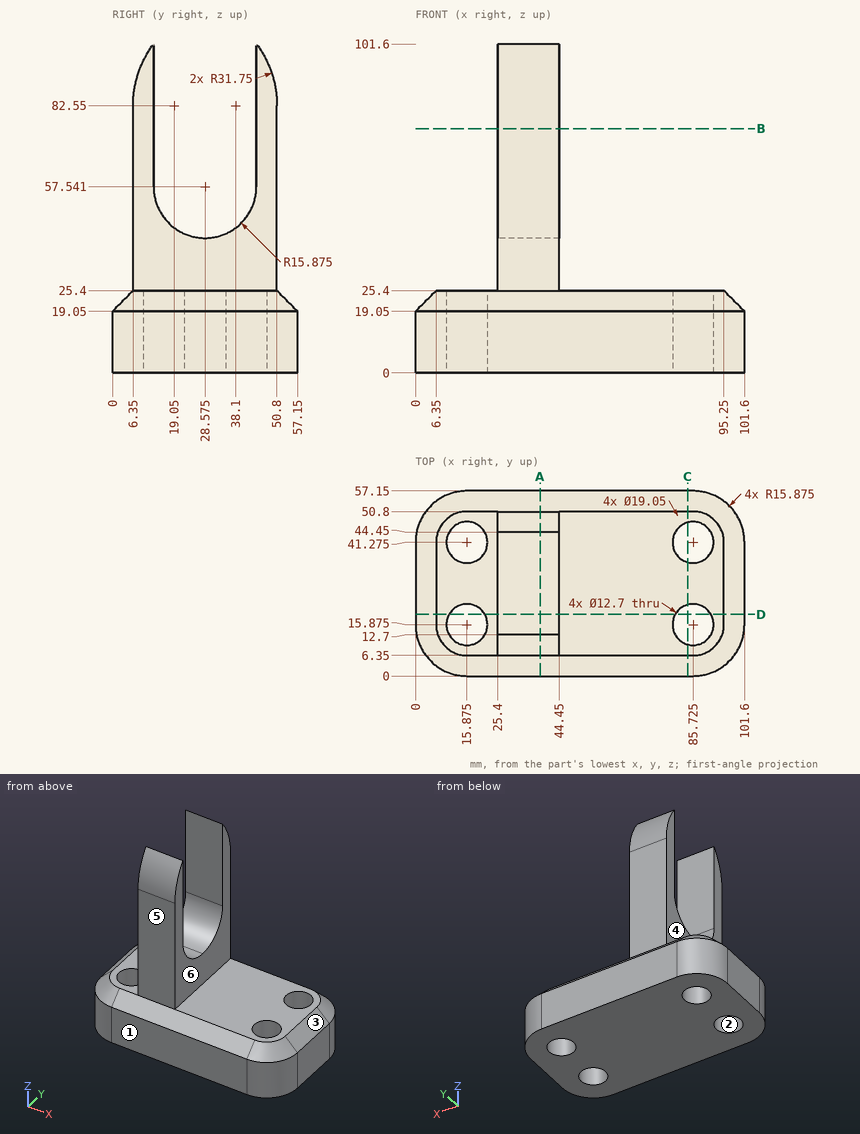
Can you work these out from the drawing? Everything is in mm from the part's minimum corner. A direction names the side the tool comes from. Round coordinates to 2 decimals unless told otherwise and drop trailing zeros. Write each loop counter-clockwise with the first axis right and the second up, starting at its lowest first coordinate (ties: lowest second). Pieces come first, ordered by that corner, then holes. Notation, with made-up numbers: M 87.5,64.5 L 93.5,64.5 A19 ccw 93.5,79.5 Z; hole C 24.5,59.25 d5. An arc over 180 degrees is marked long. Use a Markdown table: item, result.
Item 1: I want a section at B-B (z = 75.5). List the corners of the cut face in (x, y) for me.
Found:
| item | result |
|---|---|
| outline | M 25.4,6.35 L 44.45,6.35 L 44.45,12.7 L 25.4,12.7 Z; M 25.4,44.45 L 44.45,44.45 L 44.45,50.8 L 25.4,50.8 Z |
Item 2: I want a section at C-C (x = 84). List the corners of the cut face in (y, z) for me.
Found:
| item | result |
|---|---|
| outline | M 0,0 L 9.76,0 L 9.76,25.4 L 6.35,25.4 L 0,19.05 Z; M 21.99,0 L 35.16,0 L 35.16,25.4 L 21.99,25.4 Z; M 47.39,0 L 57.15,0 L 57.15,19.05 L 50.8,25.4 L 47.39,25.4 Z |
Item 3: We'd pull the mould along X, two halves only. Please class the marked faces 1, 2 and 3: released by +X, released by -X, zero draft, split by the parting line, or undercut.
Found:
| item | result |
|---|---|
| face 1 | zero draft |
| face 2 | undercut |
| face 3 | released by +X |
Item 4: I want a section at D-D (y = 19). List the corners of the cut face in (x, z) for me, and give its area (3 significant figures).
Found:
| item | result |
|---|---|
| outline | M 0,0 L 10.35,0 L 10.35,25.4 L 6.35,25.4 L 0,19.05 Z; M 21.4,0 L 80.2,0 L 80.2,25.4 L 44.45,25.4 L 44.45,44.88 L 25.4,44.88 L 25.4,25.4 L 21.4,25.4 Z; M 91.25,0 L 101.6,0 L 101.6,19.05 L 95.25,25.4 L 91.25,25.4 Z |
| area | 2,350 mm2 |
Item 5: I want a section at A-A (x = 38.5). List the corners of the cut face in (y, z) for me (3 decimals), and give its area (3 significant figures).
Found:
| item | result |
|---|---|
| outline | M 0,0 L 57.15,0 L 57.15,19.05 L 50.8,25.4 L 50.8,82.55 A31.75 ccw 44.45,101.6 L 44.45,57.541 A15.875 cw 12.7,57.541 L 12.7,101.6 A31.75 ccw 6.35,82.55 L 6.35,25.4 L 0,19.05 Z |
| area | 2,930 mm2 |
Item 6: If I drill on line 1 along X through (y, z) = (10, 36); line 2 along Z through (x, y) = (22.5, 31.5); line 3 along Y through (x, z) = (44, 75.5), over which ranges is the centre line in solid material (lowest first)? Write a range as [from, to].
Found:
| item | result |
|---|---|
| line 1 | x = [25.4, 44.45] |
| line 2 | z = [0, 25.4] |
| line 3 | y = [6.35, 12.7], [44.45, 50.8] |
Item 7: Which directions (+Z, -Z, +X, -X, +Y, -Y) give clear straight access to the entire face, cutting with the end or side of a thin tool? Please do the marked faces 4, 5 and 6.
Found:
| item | result |
|---|---|
| face 4 | +Z, -X, +Y, -Y |
| face 5 | +Z, +X, -X, -Y |
| face 6 | +Z, +X, +Y, -Y |
Item 8: For pin 1 Ø5 at (x, y) = (20, 41.5) entering from +Z; pin 2 Ø5.5 at (x, z) = (36.5, 57) entering from -Y; pin 3 Ø21 at (x, z) = (38.5, 80) entering from +Y, each with a flat end and sliding along its axis, tell me the tip position at first contact or that it passes through.
Found:
| item | result |
|---|---|
| pin 1 | stops at z = 25.4 |
| pin 2 | stops at y = 6.35 |
| pin 3 | stops at y = 50.8 |
